CAD build for the part. Positions are in the model's coordinates, mm. Face numbers are marked on the shaded views. A direction names the side the tool comes from. Coordinates: 2 decimals unless noted, no trailing zeros. Write each loop counter-clockwise with the first axis right and the second up, starting at its lowest first coordinate (ties: lowest second). Pieces come first, ordered by that corner, then holes.
```python
from build123d import *

# Parameters (mm, degrees)
ESBO_O1_R                = 1.5
RESSALTO_EXTRUS_O1_DEPTH = 3.6
FILETE1_R                = 3
FILETE2_R                = 5


with BuildPart() as part:
    # Esboço1 → Ressalto-extrusão1 (new body)
    with BuildSketch(Plane(origin=(0, 0, 0), x_dir=(0, 0, -1), z_dir=(1, 0, 0))):
        Polygon((0, 0), (20, 0), (20, 4), (15.1, 4), (15.1, 30), (4.9, 30), (4.9, 4), (0, 4), align=None)
        with Locations((10, 26.9)):
            Circle(ESBO_O1_R, mode=Mode.SUBTRACT)
        with Locations((10, 9.5)):
            Circle(ESBO_O1_R, mode=Mode.SUBTRACT)
    extrude(amount=RESSALTO_EXTRUS_O1_DEPTH)

    # Filete1
    filete1_edges = [part.edges().sort_by_distance(p)[0] for p in [
        (1.8, 30, -4.9),
        (1.8, 30, -15.1),
    ]]
    fillet(filete1_edges, radius=FILETE1_R)

    # Filete2
    # the kernel refuses this fillet: 5 mm, written as the material it takes off along each edge
    with BuildSketch(Plane(origin=(-12.247448714, 0, 0), x_dir=(0, 0, -1), z_dir=(1, 0, 0))) as filete2_piece_1:
        with BuildLine():
            CenterArc((4.898979486, 5), FILETE2_R, 191.536959033, 78.463040967)
            Line((0, 4), (-0.09797959, 3.98))
            ThreePointArc((-0.09797959, 3.98), (-0.1, 2), (-0.1, 0))
            Line((-0.1, 0), (0, -0.1))
            Line((0, -0.1), (4.898979486, -0.1))
            Line((4.898979486, -0.1), (4.898979486, 0))
        make_face()
    extrude(amount=28.094897428, mode=Mode.SUBTRACT)
    with BuildSketch(Plane(origin=(-12.247448714, 0, -20), x_dir=(0, 1.0, 1.5667467323505199e-12), z_dir=(1, 0, 0))) as filete2_piece_2:
        with BuildLine():
            CenterArc((5, 4.898979486), FILETE2_R, 180, 78.463040967)
            Line((0, 4.898979486), (-0.1, 4.898979486))
            Line((-0.1, 4.898979486), (-0.1, 0))
            Line((-0.1, 0), (0, -0.1))
            ThreePointArc((0, -0.1), (2, -0.1), (3.98, -0.09797959))
            Line((3.98, -0.09797959), (4, 0))
        make_face()
    extrude(amount=28.094897428, mode=Mode.SUBTRACT)


solid = part.part
```
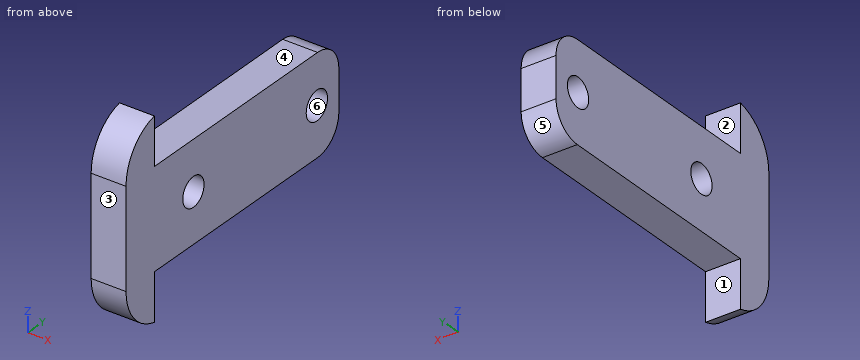
Item 1: Saw through at A-A, the plane z = -10. Write the cut outline in (x, y), and give its area (3 significant figures).
Item 2: Saw through at D-D, the plane z = -5.5. Write the cut outline in (x, y), and give its area (3 significant figures).
Item 3: Saw through at B-B, the plane y = 9.5. Write the cut outline in (x, z).
Item 4: Saw through at C-C, the plane x = 3.25. Write the cut outline in (y, z).
Item 5: Two-plate mould, pull along Z, no slides. Class the marked faces 4, 5 and 6: +Z half, -Z half, draft (parallel to the pull), parting line (faces both ways), or undercut.
Item 6: Wall check: line 1 along Y through (x, z) = (1.95, -10); line 2 along Z through (x, y) = (2.1, 27); line 3 along Z through (x, y) = (1.75, 15). Give the ranges that are in metal, low to high.
Item 7: Which spindle directions (+Z, -Z, +X, -X, +Y, -Y) get a long thin tool onto all of the face, cutting with end or side? Do the marked faces 1, 2 and 3. Say none if no direction does.
Item 8: Flat gauge pins, fed straight in: pin 1 Ø1.8 at (x, z) = (1.5, -17.5) entering from +Y; pin 2 Ø5 at (y, z) = (9.5, -10) entering from +X; pin 3 Ø1 at (x, y) = (2.5, 18) entering from -Z; pin 4 Ø1.5 at (x, z) = (1, -13) entering from +Y. Where does each tip first touch, or does it go through?
Working result:
1. outline: (0, 0) - (3.6, 0) - (3.6, 8) - (0, 8) - close; (0, 11) - (3.6, 11) - (3.6, 25.4) - (0, 25.4) - close; (0, 28.4) - (3.6, 28.4) - (3.6, 30) - (0, 30) - close
1. area: 86.4 mm2
2. outline: (0, 0) - (3.6, 0) - (3.6, 28.8) - (0, 28.8) - close
2. area: 104 mm2
3. outline: (0, -15.1) - (3.6, -15.1) - (3.6, -11.5) - (0, -11.5) - close; (0, -8.5) - (3.6, -8.5) - (3.6, -4.9) - (0, -4.9) - close
4. outline: (0, -15.1) arc R5 ccw to (4, -20) - (4, -15.1) - (27, -15.1) arc R3 ccw to (30, -12.1) - (30, -7.9) arc R3 ccw to (27, -4.9) - (4, -4.9) - (4, 0) arc R5 ccw to (0, -4.9) - close; hole circle Ø3 at (9.5, -10); hole circle Ø3 at (26.9, -10)
5. face 4: +Z half
5. face 5: -Z half
5. face 6: undercut
6. line 1: y = 0 to 8, 11 to 25.4, 28.4 to 30
6. line 2: z = -15.1 to -11.5, -8.5 to -4.9
6. line 3: z = -15.1 to -4.9
7. face 1: -Z, +X, -X, +Y
7. face 2: +Z, +X, -X, +Y
7. face 3: +Z, -Z, +X, -X, -Y
8. pin 1: stops at y = 4
8. pin 2: stops at x = 3.6
8. pin 3: stops at z = -15.1
8. pin 4: stops at y = 30
